Geometry: final body of the model. Coordinates: model frame, mm. A direction names the side the tool comes from. Give positions to 0.01 mm unless a question says otherwise; leave off trailing zeros. Loops run counter-clockwise (first coordinate to the right, second up) from the corner with the lowest first, then second, coordinate; pieces in that order, holes last.
1. Access query for faces 5 (the face through (13.6, -10.75, 8.5)), 6 (the face through (6, -16.25, 7)). Directions: +Z, -Z, +X, -X, +Y, -Y. A direction counts if a zero-diameter tool reaches every point of the face in a straight line with its end or side. Return the directions, or none.
2. Section C-C, the plane y = 3.75. Output: boundary loops of the cut face in (x, z), then the cut area to 3 significant figures.
3. First-contact query: P1, Ø1.5, axis at x = 10.5, y = 11.5, coming from the -Z side; P2, Ø3.5, axis at x = 14.5, z = 3.5, coming from the +Y side; P3, Ø2, axis at y = -6, z = 6.5, coming from the +X side. Flat tips, straight axial feed; report the tip coordinate or a pass-through.
4. Section D-D, the plane z = 1.5. Output: boundary loops of the cut face in (x, y), then the cut area to 3 significant figures.
5. Section B-B, the plane x = 0. Output: boundary loops of the cut face in (y, z).
6. Material intervals for line 1 along Y through (x, z) = (0, 3.5); line 2 along Y through (x, z) = (11, 2); line 3 along X through (y, z) = (3, 3.5), sorted ascending.
7. Draft query along Z for faces 1 (the face through (0, -3, 14)), 2 (the face through (21, -13, 7)), 3 (the face through (0, -3, 0)), 4 (the face through (19, -13, 7)). Return one class per face: +Z half, -Z half, draft (parallel to the pull), parting line (faces both ways), or undercut.
8. Section A-A, the plane z = 6.5. Output: boundary loops of the cut face in (x, y).
from build123d import *

# Parameters (mm, degrees)
SKETCH_1_R          = 4
EXTRUDE_1_DEPTH     = 14
SKETCH_2_R          = 2.75
CUT_EXTRUDE_1_DEPTH = 14
SKETCH_3_W          = 12
SKETCH_3_H          = 14
CUT_EXTRUDE_2_DEPTH = 10


with BuildPart() as part:
    # 草图1 → 凸台-拉伸1 (new body)
    with BuildSketch(Plane.XY):
        Polygon((-21, -10.75), (-9, -10.75), (-9, 16.25), (9, 16.25), (9, -10.75), (21, -10.75), (21, -16.25), (-21, -16.25), align=None)
        with Locations((0, 3.75)):
            Circle(SKETCH_1_R, mode=Mode.SUBTRACT)
    extrude(amount=EXTRUDE_1_DEPTH)

    # 草图2 → 切除-拉伸1 (cut)
    with BuildSketch(Plane(origin=(0, -10.75, 0), x_dir=(1, 0, 0), z_dir=(0, 1, 0))):
        with Locations(Location((-16.25, -7, 0), (0, 0, 270))):
            Circle(SKETCH_2_R)
        with Locations(Location((16.25, -7, 0), (0, 0, 270))):
            Circle(SKETCH_2_R)
    extrude(amount=-CUT_EXTRUDE_1_DEPTH, mode=Mode.SUBTRACT)

    # 草图3 → 切除-拉伸2 (cut)
    with BuildSketch(Plane(origin=(0, -10.75, 0), x_dir=(1, 0, 0), z_dir=(0, 1, 0))):
        with Locations((-15, -7)):
            Rectangle(SKETCH_3_W, SKETCH_3_H)
    extrude(amount=-CUT_EXTRUDE_2_DEPTH, mode=Mode.SUBTRACT)


solid = part.part
Answers below:
1. face 5: +Z, -Z, +X, +Y
1. face 6: +Z, -Z, +X, -X, -Y
2. outline: (-9, 0) - (-4, 0) - (-4, 14) - (-9, 14) - close; (4, 0) - (9, 0) - (9, 14) - (4, 14) - close
2. area: 140 mm2
3. P1: passes through
3. P2: stops at y = -10.75
3. P3: stops at x = 9
4. outline: (-9, -16.25) - (21, -16.25) - (21, -10.75) - (9, -10.75) - (9, 16.25) - (-9, 16.25) - close; hole circle Ø8 at (0, 3.75)
4. area: 601 mm2
5. outline: (-16.25, 0) - (-0.25, 0) - (-0.25, 14) - (-16.25, 14) - close; (7.75, 0) - (16.25, 0) - (16.25, 14) - (7.75, 14) - close
6. line 1: y = -16.25 to -0.25, 7.75 to 16.25
6. line 2: y = -16.25 to -10.75
6. line 3: x = -9 to -3.93, 3.93 to 9
7. face 1: +Z half
7. face 2: draft
7. face 3: -Z half
7. face 4: undercut
8. outline: (-9, -16.25) - (13.55, -16.25) - (13.55, -10.75) - (9, -10.75) - (9, 16.25) - (-9, 16.25) - close; (18.95, -16.25) - (21, -16.25) - (21, -10.75) - (18.95, -10.75) - close; hole circle Ø8 at (0, 3.75)
